Can you work these out from the model? Positions are in its coordinate system, mm. A direction names the side the tool comes from. Give positions to 0.01 mm unless a question says otherwise; leave off trailing zeros. Order: outer loops, then holes, each group sorted by start corner. A loop starts at its lowest first (then second) coordinate and runs counter-clockwise, first axis right, second up. Notation, with made-up numbers: (4, 43.25) - (15, 43.25) arc R18 ccw to (15, 70.25) - close; hole circle Ø9 at (-20, 42). An arc over 180 degrees is marked (long way). Return JSON: item names as keys, results as strings.
```python
from build123d import *

# Parameters (mm, degrees)
BOSS_EXTRUDE1_DEPTH      = 28.702
SKETCH9_R                = 8.001
SKETCH9_R_2              = 6.35
BOSS_EXTRUDE2_DEPTH      = 3.302
SKETCH16_R               = 6.35
BOSS_EXTRUDE3_DEPTH      = 12.7
CHAMFER1_SIZE            = 0.762
CHAMFER1_OF_MIRROR1_SIZE = 0.762
SKETCH17_R               = 1.27
CUT_EXTRUDE1_DEPTH       = 4.572
CIRPATTERN1_COUNT        = 5


with BuildPart() as part:
    # Sketch1 → Boss-Extrude1 (new body)
    with BuildSketch(Plane(origin=(0, 0, 0), x_dir=(0, 0, -1), z_dir=(1, 0, 0))):
        with BuildLine():
            Line((0, 15.718274541), (0, 25.4))
            ThreePointArc((0, 25.4), (-2.655022967, 25.260856142), (-5.280956947, 24.844949059))
            Line((-5.280956947, 24.844949059), (-11.061817414, 7.053289967))
            ThreePointArc((-11.061817414, 7.053289967), (-12.577998446, 5.198746045), (-14.948967427, 4.857213955))
            Line((-14.948967427, 4.857213955), (-24.156835514, 7.849031657))
            ThreePointArc((-24.156835514, 7.849031657), (-24.844949059, 5.280956947), (-25.260856142, 2.655022967))
            Line((-25.260856142, 2.655022967), (-10.126366954, -8.340827068))
            ThreePointArc((-10.126366954, -8.340827068), (-8.831116578, -10.355886507), (-9.238969967, -12.716351226))
            Line((-9.238969967, -12.716351226), (-14.929745408, -20.549031657))
            ThreePointArc((-14.929745408, -20.549031657), (-12.7, -21.997045256), (-10.331110734, -23.204054624))
            Line((-10.331110734, -23.204054624), (4.803378454, -12.208204589))
            ThreePointArc((4.803378454, -12.208204589), (7.120068242, -11.59903589), (9.238969967, -12.716351226))
            Line((9.238969967, -12.716351226), (14.929745408, -20.549031657))
            ThreePointArc((14.929745408, -20.549031657), (16.995917402, -18.875878567), (18.875878567, -16.995917402))
            Line((18.875878567, -16.995917402), (13.095018099, 0.79574169))
            ThreePointArc((13.095018099, 0.79574169), (13.231560754, 3.18728809), (14.948967427, 4.857213955))
            Line((14.948967427, 4.857213955), (24.156835514, 7.849031657))
            ThreePointArc((24.156835514, 7.849031657), (23.204054624, 10.331110734), (21.997045256, 12.7))
            Line((21.997045256, 12.7), (3.289787814, 12.7))
            ThreePointArc((3.289787814, 12.7), (1.057486028, 13.568888261), (0, 15.718274541))
        make_face()
    extrude(amount=BOSS_EXTRUDE1_DEPTH)

    # Sketch9 → Boss-Extrude2 (add)
    with BuildSketch(Plane(origin=(28.702, 0, 0), x_dir=(0, 0, -1), z_dir=(1, 0, 0))):
        Circle(SKETCH9_R)
        Circle(SKETCH9_R_2, mode=Mode.SUBTRACT)
    boss_extrude2 = extrude(amount=BOSS_EXTRUDE2_DEPTH)

    # Sketch16 → Boss-Extrude3 (add)
    with BuildSketch(Plane(origin=(28.702, 0, 0), x_dir=(0, 0, -1), z_dir=(1, 0, 0))):
        Circle(SKETCH16_R)
    boss_extrude3 = extrude(amount=BOSS_EXTRUDE3_DEPTH)

    # Chamfer1
    chamfer1_edges = [part.edges().sort_by_distance(p)[0] for p in [
        (41.402, 0, 6.35),
    ]]
    chamfer(chamfer1_edges, length=CHAMFER1_SIZE)

    # Mirror1: Boss-Extrude2, Boss-Extrude3 across plane
    add(boss_extrude2.mirror(Plane(origin=(14.351, 0, 0), x_dir=(0, 0, 1), z_dir=(1, 0, 0))))
    add(boss_extrude3.mirror(Plane(origin=(14.351, 0, 0), x_dir=(0, 0, 1), z_dir=(1, 0, 0))))

    # Chamfer1 of Mirror1
    chamfer1_of_mirror1_edges = [part.edges().sort_by_distance(p)[0] for p in [
        (-12.7, 0, 6.35),
    ]]
    chamfer(chamfer1_of_mirror1_edges, length=CHAMFER1_OF_MIRROR1_SIZE)

    # Sketch17 → Cut-Extrude1 (cut)
    with BuildSketch(Plane(origin=(0, 0, 0), x_dir=(-1, 0, 0), z_dir=(0, 0, -1))):
        with Locations((-20.828, 20.32)):
            Circle(SKETCH17_R)
        with Locations((-7.874, 20.32)):
            Circle(SKETCH17_R)
    cut_extrude1 = extrude(amount=-CUT_EXTRUDE1_DEPTH, mode=Mode.SUBTRACT)

    # CirPattern1: Cut-Extrude1 ×5 about axis
    cirpattern1_axis = Axis((0, 0, 0), (1, 0, 0))
    for i in range(1, CIRPATTERN1_COUNT):
        add(cut_extrude1.rotate(cirpattern1_axis, i * 360 / CIRPATTERN1_COUNT), mode=Mode.SUBTRACT)


solid = part.part
```
1. On a 3-axis mill with a long thin cutter (end or side, diameter ignored), from which of +Z, -Z, +X, -X, +Y, -Y can I reach the whole of each face in a straight line? I mean faces 1 (the face through (7.89, 1.94, 20.76)), 2 (the face through (14, 5, 13)), 3 (the face through (36.26, -6.2, 1.38)), 4 (the face through (14.15, -8.225, -16.026)). Say none if no direction works.
Checks:
{"face 1": "none", "face 2": "+X, -X, +Y", "face 3": "+X", "face 4": "-Z, +X, -X"}
2. For pin 1 Ø1 at (x, z) = (18.5, -13) entering from +Y; pin 2 Ø3 at (x, y) = (-5, -6) entering from +Z; pin 3 Ø1.5 at (x, y) = (27, -7.5) entering from +Z, each with a flat end and sliding along its axis, tell me the tip position at first contact or that it passes through.
Checks:
{"pin 1": "y = 12.7", "pin 2": "z = 4.48", "pin 3": "z = 12.32"}
3. Suppose I cut it at A-A (x = 15.5). List the corners of the cut face in (y, z) for me, plus the area to 3 significant figures.
Checks:
{"outline": "(-23.2, 10.33) - (-12.21, -4.8) arc R3.3 cw to (-12.72, -9.24) - (-20.55, -14.93) arc R25.4 ccw to (-17, -18.88) - (0.8, -13.1) arc R3.3 cw to (4.86, -14.95) - (7.85, -24.16) arc R25.4 ccw to (12.7, -22) - (12.7, -3.29) arc R3.3 cw to (15.72, 0) - (25.4, 0) arc R25.4 ccw to (24.84, 5.28) - (7.05, 11.06) arc R3.3 cw to (4.86, 14.95) - (7.85, 24.16) arc R25.4 ccw to (2.66, 25.26) - (-8.34, 10.13) arc R3.3 cw to (-12.72, 9.24) - (-20.55, 14.93) arc R25.4 ccw to start", "area": "1,050 mm^2"}
4. Suppose I cut it at D-D (z = -14). State how many separate pieces and enclosed holes the cut face has, plus the area to 3 significant figures.
Checks:
{"separate pieces": "2", "enclosed holes": "2", "area": "726 mm^2"}
5. If I drill on L1, parallel to Y at x = 18, z = -7; L2, parallel to Y at x = 15, z = -19.5; L3, parallel to Z at x = 13.5, y = -13, over which ranges is the centre line in solid material (lowest first)? Write a range as [from, to].
Checks:
{"L1": "[-11.59, 12.7]", "L2": "[6.34, 12.7]", "L3": "[-17.58, -9.45], [-3.71, 9.45]"}
6. Thinking about a two-plate mould opening in X: for faces 5 (the face through (28.702, 7, -5)), 6 (the face through (14.15, 5.317, 24.837)), 7 (the face through (8.81, 8.688, -19.445)), which applies, +X half, -X half, draft (parallel to the pull), parting line (faces both ways), or undercut?
Checks:
{"face 5": "+X half", "face 6": "draft", "face 7": "undercut"}
7. Suppose I cut it at C-C (y = 20.32). List the corners of the cut face in (x, z) for me, plus the area to 3 significant figures.
Checks:
{"outline": "(0, 0) - (6.6, 0) - (6.6, 4.57) - (9.14, 4.57) - (9.14, 0) - (19.56, 0) - (19.56, 4.57) - (22.1, 4.57) - (22.1, 0) - (28.7, 0) - (28.7, 6.75) - (0, 6.75) - close", "area": "171 mm^2"}
8. Suppose I cut it at B-B (z = 13.5). List the corners of the cut face in (x, y) for me.
Checks:
{"outline": "(0, -21.52) - (28.7, -21.52) - (28.7, -18.58) - (0, -18.58) - close; (0, -5.89) - (28.7, -5.89) - (28.7, 4.85) - (0, 4.85) - close"}
